```python
from build123d import *

# Parameters (mm, degrees)
F0_W     = 76.2
F0_H     = 76.2
F1_DEPTH = 76.2
F2_R     = 12.7
F3_R     = 10.16
F4_DEPTH = 76.201
F5_R     = 10.16
F6_DEPTH = 76.201
F7_R     = 10.16
F8_DEPTH = 76.201


with BuildPart() as f1:
    # F0 (on Front) → F1 (new body)
    with BuildSketch(Plane.XZ):
        with Locations((-38.1, 38.1)):
            Rectangle(F0_W, F0_H)
    extrude(amount=F1_DEPTH)

    # F2
    f2_edges = [f1.edges().sort_by_distance(p)[0] for p in [
        (0, -38.1, 76.2),
        (-76.2, -38.1, 76.2),
        (0, -38.1, 0),
        (-76.2, -38.1, 0),
    ]]
    fillet(f2_edges, radius=F2_R)

    # F3 (on face) → F4 (cut, through all)
    with BuildSketch(Plane.XZ.offset(76.2)):
        with Locations((-38.1, 38.1)):
            Circle(F3_R)
    extrude(amount=-F4_DEPTH, mode=Mode.SUBTRACT)

    # F5 (on face) → F6 (cut, through all)
    with BuildSketch(Plane.YZ):
        with Locations((-38.1, 38.1)):
            Circle(F5_R)
    extrude(amount=-F6_DEPTH, mode=Mode.SUBTRACT)

    # F7 (on face) → F8 (cut, through all)
    with BuildSketch(Plane.XY.offset(76.2)):
        with Locations((-38.1, -38.1)):
            Circle(F7_R)
    extrude(amount=-F8_DEPTH, mode=Mode.SUBTRACT)


solid = f1.part
```
Geometry check sheet. Reference: the model listing, model coordinates, mm. Give positions to 0.01 mm unless a question says otherwise; leave off trailing zeros. Write each loop counter-clockwise with the first axis right and the second up, starting at its lowest first coordinate (ties: lowest second). Pieces come first, ordered by that corner, then holes.
1) Section check B-B, the plane z = 38.1. Record the boundary of the cut face in (x, y).
2) Section check A-A, the plane y = -38.1. Record the boundary of the cut face in (x, z), and give its area (3 significant figures).
3) Material ranges on L1, parallel to Z at x = -38, y = -53; L2, parallel to X at y = -63.5, z = 38.1, recorded low to high.
4) Section check D-D, the plane z = 15. Record the boundary of the cut face in (x, y), and give its area (3 significant figures).
5) Section check C-C, the plane x = -38.1. Record the boundary of the cut face in (y, z).
6) Release check for a two-part mould opening along X. For faces 1 (the flat face through (-44, -29, 76.2)), 2 (the cylindrical face through (-48.25, -60.96, 38.55)), 3 (the cylindrical face through (-45.588, -31.233, 15.674)), 4 (the cylindrical face through (-3.62, -38.63, 72.38)) record: pulls with the +X half, pulls with the -X half, needs draft (parallel to the pull), parting line crosses it, or undercut.
Computed:
1. outline: (-76.2, -76.2) - (-48.26, -76.2) - (-48.26, -48.26) - (-76.2, -48.26) - close; (-76.2, -27.94) - (-48.26, -27.94) - (-48.26, 0) - (-76.2, 0) - close; (-27.94, -76.2) - (0, -76.2) - (0, -48.26) - (-27.94, -48.26) - close; (-27.94, -27.94) - (0, -27.94) - (0, 0) - (-27.94, 0) - close
2. outline: (-76.2, 12.7) arc R12.7 ccw to (-63.5, 0) - (-48.26, 0) - (-48.26, 27.94) - (-76.2, 27.94) - close; (-76.2, 48.26) - (-48.26, 48.26) - (-48.26, 76.2) - (-63.5, 76.2) arc R12.7 ccw to (-76.2, 63.5) - close; (-27.94, 0) - (-12.7, 0) arc R12.7 ccw to (0, 12.7) - (0, 27.94) - (-27.94, 27.94) - close; (-27.94, 48.26) - (0, 48.26) - (0, 63.5) arc R12.7 ccw to (-12.7, 76.2) - (-27.94, 76.2) - close
2. area: 2,980 mm2
3. L1: z = 0 to 27.94, 48.26 to 76.2
3. L2: x = -76.2 to -48.26, -27.94 to 0
4. outline: (-76.2, -76.2) - (0, -76.2) - (0, 0) - (-76.2, 0) - close; hole circle Ø20.32 at (-38.1, -38.1)
4. area: 5,480 mm2
5. outline: (-76.2, 0) - (-48.26, 0) - (-48.26, 27.94) - (-76.2, 27.94) - close; (-76.2, 48.26) - (-48.26, 48.26) - (-48.26, 76.2) - (-76.2, 76.2) - close; (-27.94, 0) - (0, 0) - (0, 27.94) - (-27.94, 27.94) - close; (-27.94, 48.26) - (0, 48.26) - (0, 76.2) - (-27.94, 76.2) - close
6. face 1: needs draft
6. face 2: undercut
6. face 3: undercut
6. face 4: pulls with the +X half
